Verification items for the finished model (mm, model axes). A direction names the side the tool comes from. Round coordinates to 2 decimals unless told otherwise and drop trailing zeros. Order: outer loops, then holes, each group sorted by start corner. A loop starts at its lowest first (then second) coordinate and runs counter-clockwise, first axis right, second up. Notation, with made-up numbers: M 30,-27.5 L 36,-27.5 A18 ccw 36,7.5 Z; hole C -38,48.5 d7. An arc over 180 degrees is marked long. Use CSV: the item, a comma, the result in double quotes. Start each with the question number.
Q1. Sectioned sample at D-D (z = 1.5). Enter the section's corners in (x, y).
Q2. Gauge pin test, flat ends, axial feed: pin 1 Ø4.5 at (x, y) = (3, 0) entering from +Z; pin 2 Ø1.5 at (x, z) = (5.5, 3) entering from -Y; pin 3 Ø2 at (x, z) = (0, 2) entering from +Y. Record the tip position at first contact, or that the pin passes through.
Q3. Sectioned sample at A-A (y = 0). Enter the section's corners in (x, z).
Q4. Sectioned sample at B-B (z = 6). Enter the section's corners in (x, y), and give its area (4 significant figures).
Q5. Scan lines: line 1 (Y direction, x = 0, z = 3.25); line 2 (Z direction, x = -6, y = 0.25); line 3 (Y direction, x = 0, z = 6). Record each from-to range of solid material in increasing order.
Q6. Set-up check for faces 4 (the face through (-8.59, -0.38, 1.97)), 5 (the face through (0, 0, -1.5)): record each of +Z, -Z, +X, -X, +Y, -Y from which the full face is reachable in a straight line by a thin tool's end or side.
Q7. Mould release check, pull along X, two halves, no side actions. Record for faces 1 (the face through (9.252, 2.914, -0.493)), 2 (the face through (-0.92, -7.04, 3.94)), 3 (the face through (-1, -9, 0)): +X half, -X half, draft (parallel to the pull), parting line (faces both ways), or undercut.
Autodesk Inventor part; units mm, degrees
ref_plane "YZ Plane" through (0, 0, 0) normal (1, 0, 0) x (0, 1, 0)
ref_plane "XZ Plane" through (0, 0, 0) normal (0, 1, 0) x (-1, 0, 0)
ref_plane "XY Plane" through (0, 0, 0) normal (0, 0, 1) x (1, 0, 0)
sketch "Sketch1" plane through (0, 0, 0) normal (0, 0, 1) x (1, 0, 0)
  circle A0 centre (0, 0) radius 9.7
  circle A1 centre (0, 0) radius 8.6
  circle A2 centre (0, 0) radius 7.1
  dimension "d0" = 19.4
  dimension "d1" = 17.2
  dimension "d6" = 14.2
extrude "Extrusion1" add sketch "Sketch1" along normal blind 8 contours A1 | A2
extrude "Extrusion2" add sketch "Sketch1" against normal blind 1.5 contours A0 | A1 | A2
extrude "Extrusion3" cut sketch "Sketch1" along normal up to next contours A2
fillet "Fillet1" radius 0.5 1 edges at (-9.7, 0, -1.5)
chamfer "Chamfer1" distance 0.3 distance2 4 1 edges at (-8.6, 0, 8) measured on face at (7.9479, -1.2524, 8)
properties part number "Rodend19mil"
Verdict:
1,outline,"C 0,0 d17.2; hole C 0,0 d14.2"
2,pin 1,"stops at z = 0"
2,pin 2,"stops at y = -7.17"
2,pin 3,"stops at y = 8.6"
3,outline,"M -9.7,-1 A0.5 ccw -9.2,-1.5 L 9.2,-1.5 A0.5 ccw 9.7,-1 L 9.7,0 L 8.6,0 L 8.6,4 L 8.3,8 L 7.1,8 L 7.1,0 L -7.1,0 L -7.1,8 L -8.3,8 L -8.6,4 L -8.6,0 L -9.7,0 Z"
4,outline,"C 0,0 d16.9; hole C 0,0 d14.2"
4,area,"65.95 mm²"
5,line 1,"y = -8.6 to -7.1, 7.1 to 8.6"
5,line 2,"z = -1.5 to 0"
5,line 3,"y = -8.45 to -7.1, 7.1 to 8.45"
6,face 4,"+Z"
6,face 5,"-Z, +X, -X, +Y, -Y"
7,face 1,"parting line"
7,face 2,"undercut"
7,face 3,"draft"
